```python
from build123d import *

# Parameters (mm, degrees)
F0_R     = 143.65
F1_DEPTH = 12.7
F2_T     = -2.54
F4_D     = 15.875


with BuildPart() as f1:
    # F0 (on Top) → F1 (new body)
    with BuildSketch(Plane.XY):
        Circle(F0_R)
    extrude(amount=F1_DEPTH)

    # F2
    f2_openings = [f1.faces().sort_by_distance(p)[0] for p in [
        (0, 0, 0),
    ]]
    offset(amount=F2_T, openings=f2_openings)

    # F4 (through all)
    with Locations(Plane.XY.offset(12.7)):
        with Locations((0, 0)):
            Hole(F4_D / 2)


solid = f1.part
```
Input: part model. Units: mm. Frame: model coordinates. A direction names the side the tool comes from. Coordinates: 2 decimals unless noted, no trailing zeros. Write each loop counter-clockwise with the first axis right and the second up, starting at its lowest first coordinate (ties: lowest second). Pieces come first, ordered by that corner, then holes. Notation, with made-up numbers: (64, -2.75) - (113, -2.75) arc R13 ccw to (113, 11.25) - close; hole circle Ø10 at (-4, -13). An arc over 180 degrees is marked (long way). Put each result on its own line as item: value. Start each with the question number.
1) Contact query for flat-ended pins moving along their axis: pin 1 (1.5 mm diameter, centred on x = 64, y = 85.5, fed in from -Z); pin 2 (6 mm diameter, centred on x = -43.5, z = 4, fed in from +Y); pin 3 (2 mm diameter, centred on y = -35, z = 7.5, fed in from +X). Output: stop coordinate, or through.
2) Ray query, L1, parallel to Y at x = 0, z = 4.25; L2, parallel to Y at x = 0, z = 11.9; L3, parallel to Z at x = -9, y = -4.5. Return the intervals inside material, ascending.
3) Mould query, pull axis Y, two halves, no side actions, for faces 1 (the face through (-2, -29, 10.16)), 2 (the face through (-31.141, -140.234, 6.261)), 3 (the face through (30, 2, 12.7)), 4 (the face through (1.72, -7.75, 11.41)). Classes: pulls with the +Y half, pulls with the -Y half, needs draft (parallel to the pull), parting line crosses it, or undercut.
4) Reachability of faces 5 (the face through (134.594, 42.386, 5.009)), 6 (the face through (95, -106, 0)) from +Z, -Z, +X, -X, +Y, -Y: full face, straight path, thin tool, end or side. Return the list, or none.
5) Cut plane D-D (x = -41.5). Return the cut outline in (y, z), plus the area to 3 significant figures.
6) Cut plane A-A (x = 0). Return the cut outline in (y, z), plus the area to 3 significant figures.
7) Cut plane C-C (z = 3.75). Return the cut outline in (x, y), plus the area to 3 significant figures.
Resolved:
1. pin 1: stops at z = 10.16
1. pin 2: stops at y = 137.82
1. pin 3: stops at x = 139.57
2. L1: y = -143.65 to -141.11, 141.11 to 143.65
2. L2: y = -143.65 to -7.94, 7.94 to 143.65
2. L3: z = 10.16 to 12.7
3. face 1: undercut
3. face 2: parting line crosses it
3. face 3: needs draft
3. face 4: undercut
4. face 5: -Z
4. face 6: -Z, +X, -X, +Y, -Y
5. outline: (-137.52, 0) - (-134.87, 0) - (-134.87, 10.16) - (134.87, 10.16) - (134.87, 0) - (137.52, 0) - (137.52, 12.7) - (-137.52, 12.7) - close
5. area: 753 mm2
6. outline: (-143.65, 0) - (-141.11, 0) - (-141.11, 10.16) - (-7.94, 10.16) - (-7.94, 12.7) - (-143.65, 12.7) - close; (7.94, 10.16) - (141.11, 10.16) - (141.11, 0) - (143.65, 0) - (143.65, 12.7) - (7.94, 12.7) - close
6. area: 741 mm2
7. outline: circle Ø287.3 at (0, 0); hole circle Ø282.22 at (0, 0)
7. area: 2,270 mm2
